Check sheet for the modelled part. Datum: model origin and axes. Units: mm. A direction names the side the tool comes from. Give positions to 0.01 mm unless a question says otherwise; leave off trailing zeros. Write each loop counter-clockwise with the first axis right and the second up, starting at its lowest first coordinate (ties: lowest second). Pieces come first, ordered by that corner, then holes. Notation, with made-up numbers: (59, 32) -> (101, 32) arc R16 ccw to (101, 39) -> close; hole circle Ø9 at (42.5, 40.5). An arc over 180 degrees is marked (long way). Answer as a JSON object with one key per item and string values.
from build123d import *

# Parameters (mm, degrees)
PAD022_DEPTH    = 14.8
POCKET021_DEPTH = 11
PAD023_DEPTH    = 14
POCKET022_DEPTH = 2
SKETCH053_R     = 0.95
POCKET023_DEPTH = 22
SKETCH054_R     = 1.65
POCKET024_DEPTH = 20
FILLET006_R     = 1
CHAMFER022_SIZE = 1
SKETCH055_R     = 0.65
POCKET025_DEPTH = 5


with BuildPart() as part:
    # Sketch049 → Pad022 (new body)
    with BuildSketch(Plane.XY.offset(2.1)):
        Polygon((0, 0), (0, 14), (-9.781659, 18.59873), (-15.64829, 23.521417), (-18.20313, 23.521417), (-18.20313, -23.478583), (-15.64829, -23.478583), (-9.796058, -18.567977), (0, -14), align=None)
    extrude(amount=PAD022_DEPTH)

    # Sketch050 → Pocket021 (cut)
    with BuildSketch(Plane(origin=(-1, 0, 4.1), x_dir=(1, 0, 0), z_dir=(0, 0, 1))):
        Polygon((0, 0), (0, 12), (-9.697087, 16.558969), (-11.439745, 18.021232), (-25.20447, 18.021232), (-25.20447, -17.978768), (-11.439745, -17.978768), (-9.711362, -16.528482), (0, -12), align=None)
    extrude(amount=POCKET021_DEPTH, mode=Mode.SUBTRACT)

    # Sketch051 → Pad023 (join)
    with BuildSketch(Plane(origin=(-1, 0, 7.2), x_dir=(0, 1, 0), z_dir=(1, 0, 0))):
        Polygon((-14.4, 0), (-14.4, 2.5), (-9.1, 2.5), (-9.1, 1), (-11.4, 1), (-11.4, -1), (-9.1, -1), (-9.1, -2.5), (-14.4, -2.5), align=None)
        Polygon((9.1, 1), (11.4, 1), (11.4, 0), (11.4, -1), (9.1, -1), (9.1, -2.5), (14.4, -2.5), (14.4, 2.5), (9.1, 2.5), align=None)
    extrude(amount=-PAD023_DEPTH)

    # Sketch052 → Pocket022 (cut)
    with BuildSketch(Plane(origin=(0, 0, 9.7), x_dir=(0, 1, 0), z_dir=(1, 0, 0))):
        with BuildLine():
            Line((-3.53, 1.9), (3.37, 1.9))
            ThreePointArc((4.8, 0.7), (4.268438, 1.518597), (3.37, 1.9))
            Line((4.8, -0.7), (4.8, 0.7))
            ThreePointArc((3.45, -1.9), (4.308438, -1.506368), (4.8, -0.7))
            Line((-3.45, -1.9), (3.45, -1.9))
            ThreePointArc((-4.8, -0.6), (-4.323725, -1.456368), (-3.45, -1.9))
            Line((-4.8, -0.6), (-4.8, 0.8))
            ThreePointArc((-3.53, 1.9), (-4.333152, 1.544139), (-4.8, 0.8))
        make_face()
    extrude(amount=-POCKET022_DEPTH, mode=Mode.SUBTRACT)

    # Sketch053 → Pocket023 (cut)
    with BuildSketch(Plane.YZ):
        with Locations((-21.7, 9.5)):
            Circle(SKETCH053_R)
        with Locations((21.7, 9.5)):
            Circle(SKETCH053_R)
    extrude(amount=-POCKET023_DEPTH, mode=Mode.SUBTRACT)

    # Sketch054 → Pocket024 (cut)
    with BuildSketch(Plane.YZ.offset(3)):
        with Locations((-21.7, 9.5)):
            Circle(SKETCH054_R)
        with Locations((21.7, 9.5)):
            Circle(SKETCH054_R)
    extrude(amount=-POCKET024_DEPTH, mode=Mode.SUBTRACT)

    # Fillet006
    fillet006_edges = [part.edges().sort_by_distance(p)[0] for p in [
        (0, -14, 9.5),
        (0, 14, 9.5),
    ]]
    fillet(fillet006_edges, radius=FILLET006_R)

    # Chamfer022
    chamfer022_edges = [part.edges().sort_by_distance(p)[0] for p in [
        (-12.714975, 21.060074, 2.1),
        (-16.92571, 23.521417, 2.1),
        (-5.178098, 16.434421, 2.1),
        (0, 6.682568, 2.1),
        (-0.155766, 13.90111, 2.1),
        (0, -6.681465, 2.1),
        (-12.722174, -21.02328, 2.1),
        (-16.92571, -23.478583, 2.1),
        (-5.18672, -16.418607, 2.1),
        (-0.156609, -13.900229, 2.1),
        (-16.92571, -23.478583, 16.9),
        (-12.722174, -21.02328, 16.9),
        (-5.18672, -16.418607, 16.9),
        (-0.156609, -13.900229, 16.9),
        (0, -6.681465, 16.9),
        (0, 6.682568, 16.9),
        (-5.178098, 16.434421, 16.9),
        (-0.155766, 13.90111, 16.9),
        (-12.714975, 21.060074, 16.9),
        (-16.92571, 23.521417, 16.9),
    ]]
    chamfer(chamfer022_edges, length=CHAMFER022_SIZE)

    # Sketch055 → Pocket025 (cut)
    with BuildSketch(Plane.YZ.offset(-11)):
        with Locations((-13, 7.2)):
            Circle(SKETCH055_R)
        with Locations((13, 7.2)):
            Circle(SKETCH055_R)
    extrude(amount=-POCKET025_DEPTH, mode=Mode.SUBTRACT)


with BuildPart() as part_1:
    # Body018 placement: moved
    add(part.part.moved(Location((42, 0, 0))))


solid = part_1.part
1. Sectioned sample at D-D, the plane y = 8.5. Enter the section's corners in (x, z), plus the area to 3 significant figures.
Determined:
{"outline": "(23.8, 2.1) -> (41, 2.1) -> (42, 3.1) -> (42, 15.9) -> (41, 16.9) -> (23.8, 16.9) -> (23.8, 15.1) -> (41, 15.1) -> (41, 4.1) -> (23.8, 4.1) -> close", "area": "79.2 mm^2"}
2. Sectioned sample at A-A, the plane y = 1. Enter the section's corners in (x, z).
Determined:
{"outline": "(23.8, 2.1) -> (41, 2.1) -> (42, 3.1) -> (42, 7.8) -> (41, 7.8) -> (41, 4.1) -> (23.8, 4.1) -> close; (23.8, 15.1) -> (41, 15.1) -> (41, 11.6) -> (42, 11.6) -> (42, 15.9) -> (41, 16.9) -> (23.8, 16.9) -> close"}
3. Go/stop test with flat-tipped pins: P1, Ø1.6, axis at x = 31.5, z = 9, coming from the -Y side; P2, Ø5, axis at x = 38, z = 13.5, coming from the +Y side; P3, Ø3, axis at x = 28.5, z = 13, coming from the +Y side. Record where each tip stops, or that it passes through.
Determined:
{"P1": "y = -19.83", "P2": "y = 17.06", "P3": "y = 22.98"}
4. Mould release check, pull along Z, two halves, no side actions. Record for faces 1 (the face through (41.5, -0.2, 16.4)), 2 (the face through (24.41, -22.4, 10.14)), 3 (the face through (42, 0, 7)), 4 (the face through (41.43, -13.64, 2.61)): released by +Z, released by -Z, zero draft, split by the parting line, or undercut.
Determined:
{"face 1": "released by +Z", "face 2": "undercut", "face 3": "zero draft", "face 4": "released by -Z"}
5. Sectioned sample at B-B, the plane x = 35. Enter the section's corners in (y, z), plus the area to 3 significant figures.
Determined:
{"outline": "(-17.26, 3.1) -> (-16.16, 2.1) -> (16.19, 2.1) -> (17.29, 3.1) -> (17.29, 15.9) -> (16.19, 16.9) -> (-16.16, 16.9) -> (-17.26, 15.9) -> close; (-14.4, 4.7) -> (-9.1, 4.7) -> (-9.1, 6.2) -> (-11.4, 6.2) -> (-11.4, 8.2) -> (-9.1, 8.2) -> (-9.1, 9.7) -> (-14.4, 9.7) -> close; (9.1, 4.7) -> (14.4, 4.7) -> (14.4, 9.7) -> (9.1, 9.7) -> (9.1, 8.2) -> (11.4, 8.2) -> (11.4, 6.2) -> (9.1, 6.2) -> close; hole (-14.8, 4.1) -> (14.82, 4.1) -> (14.82, 15.1) -> (-14.8, 15.1) -> close", "area": "227 mm^2"}
6. Scan lines: L1, parallel to Y at x = 27.35, z = 9.5; L2, parallel to Y at x = 27, z = 11; L3, parallel to Z at x = 29.15, y = 13. Record each from-to range of solid material in increasing order. Write a range as [from, to].
Determined:
{"L1": "[-20.05, -17.98], [-14.4, -9.1], [9.1, 14.4], [18.02, 20.05]", "L2": "[-22.93, -22.39], [-21.01, -17.98], [18.02, 21.01], [22.39, 22.98]", "L3": "[2.1, 4.1], [4.7, 6.55], [7.85, 9.7], [15.1, 16.9]"}
7. Sectioned sample at C-C, the plane x = 28.75. State how many separate pieces and enclosed holes the cut face has, plus the area to 3 significant figures.
Determined:
{"separate pieces": "3", "enclosed holes": "3", "area": "271 mm^2"}
8. Access from +Z, -Z, +X, -X, +Y, -Y to the whole of each face (thin tool, end or side, straight path). Record for faces 5 (the face through (25, -21.7, 8.4)), 6 (the face through (32, 0, 16.9)), 7 (the face through (41.507, 4.298, 8.185)), 8 (the face through (34, -11.4, 7)), 9 (the face through (41.41, -13.63, 16.41)).
Determined:
{"face 5": "+X", "face 6": "+Z, +X, -X, +Y, -Y", "face 7": "+X, -X", "face 8": "-X", "face 9": "+Z, +X, -Y"}
